Check sheet for the drawn part. Datum: minimum x, y, z corner. Units: mm. A direction names the side the tool comes from. Round coordinates to 2 decimals unless told otherwise and drop trailing zeros. Write each loop counter-clockwise with the first axis right and the second up, starting at its lowest first coordinate (ties: lowest second). Pieces come first, ordered by that corner, then holes. Notation, with made-up numbers: M 69.5,44.25 L 97.5,44.25 A17 cw 97.5,48.25 Z; hole C -4.75,31.5 d1. An arc over 180 degrees is marked long. One line per item, written item: value. Start each with the question number.
1. Depth check by flat-ended pin: P1, Ø3, axis at y = 6.35, z = 3.81, coming from the -X side; P2, Ø1, axis at x = 2.5, y = 7, coming from the -Z side; P3, Ø1.3, axis at x = 3, y = 6, coming from the +Z side. Enter the tip coordinate at first touch or a pass-through.
2. Access from +Z, -Z, +X, -X, +Y, -Y to the whole of each face (thin tool, end or side, straight path). Record for the marked faces 4, 5, 6, 7 and 8.
3. Scan lines: probe 1 along Y at (x, z) = (1.6, 3.81); probe 2 along X at (y, z) = (9, 6.25); probe 3 along Z at (x, y) = (1.85, 5.75) (1 decimal). Record each from-to range of solid material in increasing order. Write a range as [from, to].
4. Release check for a two-part mould opening along Y. For the marked faces 1, 2 and 3 record: pulls with the +Y half, pulls with the -Y half, needs draft (parallel to the pull), parting line crosses it, or undercut.
5. Section check A-A (z = 3.81). Record the boundary of the cut face in (x, y).
6. Section check D-D (z = 6). Record the boundary of the cut face in (x, y).
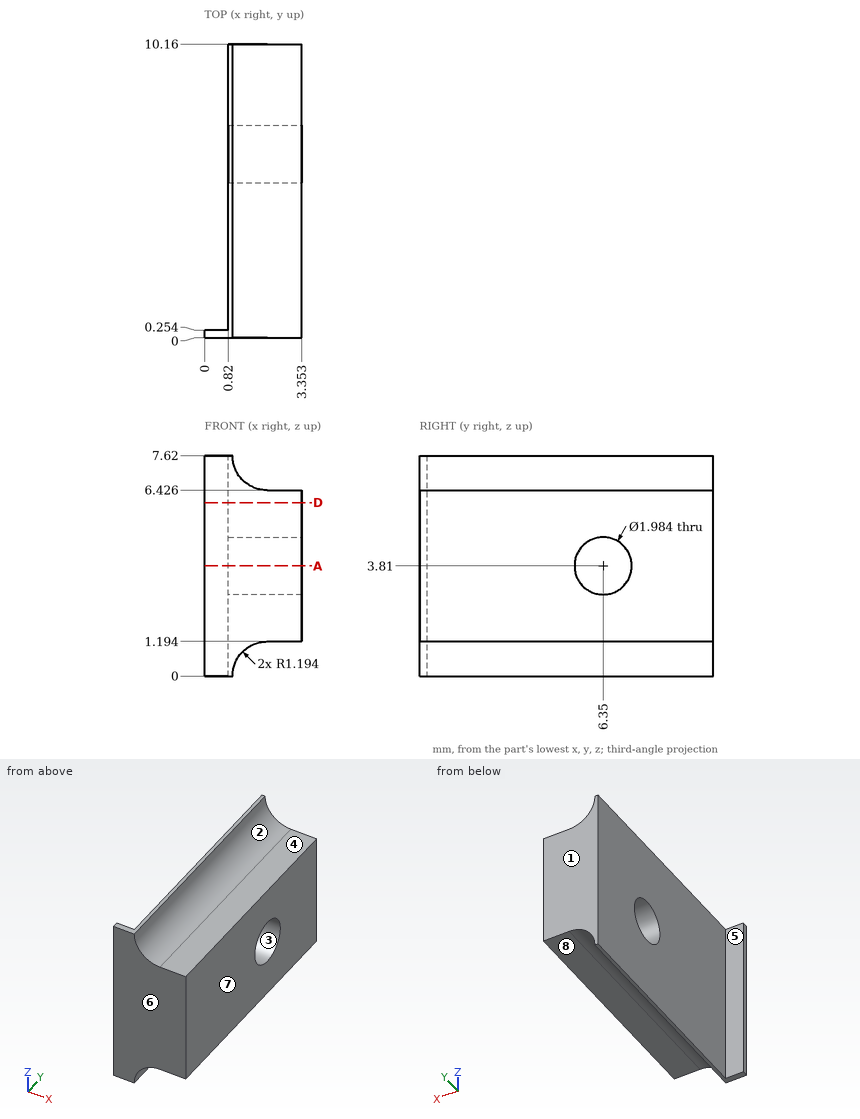
Result sheet:
1. P1: stops at x = 0.82
1. P2: stops at z = 1.18
1. P3: stops at z = 6.43
2. face 4: +Z, +X, +Y, -Y
2. face 5: +Z, -Z, -X, +Y
2. face 6: +Z, -Z, +X, -X, -Y
2. face 7: +Z, -Z, +X, +Y, -Y
2. face 8: -Z, +X, +Y, -Y
3. probe 1: y = [0, 5.36], [7.34, 10.16]
3. probe 2: x = [0.82, 3.35]
3. probe 3: z = [1.2, 3], [4.6, 6.5]
4. face 1: pulls with the +Y half
4. face 2: needs draft
4. face 3: undercut
5. outline: M 0,0 L 3.35,0 L 3.35,5.36 L 0.82,5.36 L 0.82,0.25 L 0,0.25 Z; M 0.82,7.34 L 3.35,7.34 L 3.35,10.16 L 0.82,10.16 Z
6. outline: M 0,0 L 3.35,0 L 3.35,10.16 L 0.82,10.16 L 0.82,0.25 L 0,0.25 Z
